```python
from build123d import *

# Parameters (mm, degrees)
F1_DEPTH = 1.5
F2_W     = 3.3
F2_H     = 4
F2_W_2   = 17
F2_H_2   = 6
F3_DEPTH = 0.5
F4_W     = 23
F4_H     = 2
F5_DEPTH = 0.3


with BuildPart() as f1:
    # F0 (on Top) → F1 (new body)
    with BuildSketch(Plane.XY):
        Polygon((0, 11), (0, 0), (40, 0), (40, 11), (36.7, 11), (36.7, 2), (3.3, 2), (3.3, 11), align=None)
    extrude(amount=F1_DEPTH)

    # F2 (on face) → F3 (cut)
    with BuildSketch(Plane.XY.offset(1.5)):
        with Locations((38.35, 4)):
            Rectangle(F2_W, F2_H)
        with Locations((8.5, 3)):
            Rectangle(F2_W_2, F2_H_2)
    extrude(amount=-F3_DEPTH, mode=Mode.SUBTRACT)

    # F4 (on face) → F5 (join)
    with BuildSketch(Plane.XY.offset(1.5)):
        with Locations((28.5, 1)):
            Rectangle(F4_W, F4_H)
    extrude(amount=F5_DEPTH)


solid = f1.part
```
CAD build for the part. Positions are in the model's coordinates, mm. A direction names the side the tool comes from. Round coordinates to 2 decimals unless told otherwise and drop trailing zeros. Loops run counter-clockwise (first coordinate to the right, second up) from the corner with the lowest first, then second, coordinate; pieces in that order, holes last. Notation, with made-up numbers: (-39.5, -1.5) - (-20.5, -1.5) arc R17 cw to (-20.5, 31.5) - close; hole circle Ø4 at (-26, -29.5). An arc over 180 degrees is marked (long way). Return JSON: item names as keys, results as strings. Group by question number.
Q1. Band-saw the part on C-C on x = 35. Give the cut face in (y, z).
Q2. Tool access for faces 1 (the face through (6.5, 1.7, 1)), 2 (the face through (38, 11, 1)), 3 (the face through (3.3, 6.4, 0.6)), 4 (the face through (38, 9, 1.5)), 5 (the face through (20, 1, 0)): list every direction of +Z, -Z, +X, -X, +Y, -Y with a clear straight run to the whole face (end or side of a thin tool).
Q3. Band-saw the part on B-B on x = 9. Give the cut face in (y, z).
Q4. Flat gauge pins, fed straight in: pin 1 Ø1 at (x, y) = (39, 4.5) entering from +Z; pin 2 Ø0.5 at (x, z) = (17.5, 1) entering from +Y; pin 3 Ø1.6 at (x, y) = (37.5, 8.5) entering from +Z. Where does each tip first touch, or does it go through?
Q5. Two-plate mould, pull along X, no slides. Class faces 6 (the face through (38, 4, 1)), 7 (the face through (21, 2, 1)), 8 (the face through (0, 5.6, 0.6)): +X half, -X half, draft (parallel to the pull), parting line (faces both ways), or undercut.
Q6. Band-saw the part on A-A on y = 8.25. Give the cut face in (x, z).
Q7. Drill centre lines: line 1 along X through (y, z) = (10.25, 0.7); line 2 along Y through (x, z) = (13, 0.2); line 3 along Y through (x, z) = (37, 1.3). Where is each one in solid material? Low to high. Write a range as [from, to].
Solutions:
{
 "1": {"outline": "(0, 0) - (2, 0) - (2, 1.8) - (0, 1.8) - close"},
 "2": {"face 1": "+Z, -X, -Y", "face 2": "+Z, -Z, +X, -X, +Y", "face 3": "+Z, -Z, +Y", "face 4": "+Z, +X, -X, +Y", "face 5": "-Z, +X, -X, +Y, -Y"},
 "3": {"outline": "(0, 0) - (2, 0) - (2, 1) - (0, 1) - close"},
 "4": {"pin 1": "stops at z = 1", "pin 2": "stops at y = 2", "pin 3": "stops at z = 1.5"},
 "5": {"face 6": "draft", "face 7": "undercut", "face 8": "-X half"},
 "6": {"outline": "(0, 0) - (3.3, 0) - (3.3, 1.5) - (0, 1.5) - close; (36.7, 0) - (40, 0) - (40, 1.5) - (36.7, 1.5) - close"},
 "7": {"line 1": "x = [0, 3.3], [36.7, 40]", "line 2": "y = [0, 2]", "line 3": "y = [0, 2], [6, 11]"}
}
